Here's how the part is built. I have some questions about the finished solid (model axes, mm). Give positions to 0.01 mm unless a question says otherwise; leave off trailing zeros. Put each result on its own line as item: value. Start each with the question number.
from build123d import *

# Parameters (mm, degrees)
SKETCH3_R                    = 110
BOSS_EXTRUDE_GB_BASEOD_DEPTH = 10
SKETCH4_R                    = 2.75
CUT_EXTRUDE1_DEPTH           = 156.884572681
CHAMFER1_SIZE                = 2
SKETCH7_R                    = 2.25
CUT_EXTRUDE2_DEPTH           = 156.884572681


with BuildPart() as part:
    # Sketch3 → Boss-Extrude_GB_BaseOD (new body)
    with BuildSketch(Plane(origin=(0, 0, 0), x_dir=(1, 0, 0), z_dir=(0, 1, 0))):
        with Locations(Location((0, 0, 0), (0, 0, 270))):
            Circle(SKETCH3_R)
    extrude(amount=BOSS_EXTRUDE_GB_BASEOD_DEPTH)

    # Sketch4 → Cut-Extrude1 (cut, through all)
    with BuildSketch(Plane(origin=(0, 10, 0), x_dir=(1, 0, 0), z_dir=(0, 1, 0))):
        with Locations(Location((-85, 0, 0), (0, 0, 270))):
            Circle(SKETCH4_R)
        with Locations(Location((0, 85, 0), (0, 0, 270))):
            Circle(SKETCH4_R)
        with Locations(Location((85, 0, 0), (0, 0, 270))):
            Circle(SKETCH4_R)
        with Locations(Location((0, -85, 0), (0, 0, 270))):
            Circle(SKETCH4_R)
    extrude(amount=-CUT_EXTRUDE1_DEPTH, mode=Mode.SUBTRACT)

    # Chamfer1
    chamfer1_edges = [part.edges().sort_by_distance(p)[0] for p in [
        (0, 0, -110),
        (0, 10, -110),
    ]]
    chamfer(chamfer1_edges, length=CHAMFER1_SIZE)

    # Sketch7 → Cut-Extrude2 (cut, through all)
    with BuildSketch(Plane(origin=(0, 10, 0), x_dir=(1, 0, 0), z_dir=(0, 1, 0))):
        with Locations(Location((14.849242405, 0.707106781, 0), (0, 0, 270))):
            Circle(SKETCH7_R)
        with Locations(Location((0.707106781, 14.849242405, 0), (0, 0, 90))):
            Circle(SKETCH7_R)
        with Locations(Location((-14.849242405, -0.707106781, 0), (0, 0, 270))):
            Circle(SKETCH7_R)
        with Locations(Location((-0.707106781, -14.849242405, 0), (0, 0, 90))):
            Circle(SKETCH7_R)
    extrude(amount=-CUT_EXTRUDE2_DEPTH, mode=Mode.SUBTRACT)


solid = part.part
1) I'm going to push flat-ended pins straight in: pin 1 Ø1.5 at (y, z) = (3.5, 28.5) entering from +X; pin 2 Ø4 at (y, z) = (7.5, -27) entering from +X; pin 3 Ø2 at (y, z) = (3.5, 58.5) entering from -X (3 decimals). Where does each tip first touch, or does it pass through?
2) Thinking about a two-plate mould opening in Z: for faces 1 (the cylindrical face through (0.121, 5.07, 82.253)), 2 (the flat face through (2, 0, -2)), 3 (the cylindrical face through (-97.59, 4.96, 50.76)), which applies, released by +Z, released by -Z, zero draft, split by the parting line, or undercut?
3) I want a section at A-A, the plane y = 5. State how many separate pieces and enclosed holes the cut face has, and give its area (3 significant figures).
4) I need wall thicknesses on probe 1 along X at (y, z) = (6, 0); probe 2 along X at (y, z) = (3, -83); probe 3 along Z at (x, y) = (-40.5, 5.25). Which ranges of each line are inside material? Lowest first, please.
Established:
1. pin 1: stops at x = 106.44
1. pin 2: stops at x = 107.12
1. pin 3: stops at x = -93.775
2. face 1: undercut
2. face 2: zero draft
2. face 3: split by the parting line
3. separate pieces: 1
3. enclosed holes: 8
3. area: 37,900 mm2
4. probe 1: x = -110 to -87.75, -82.25 to -16.99, -12.71 to 12.71, 16.99 to 82.25, 87.75 to 110
4. probe 2: x = -72.19 to -1.89, 1.89 to 72.19
4. probe 3: z = -102.27 to 102.27
